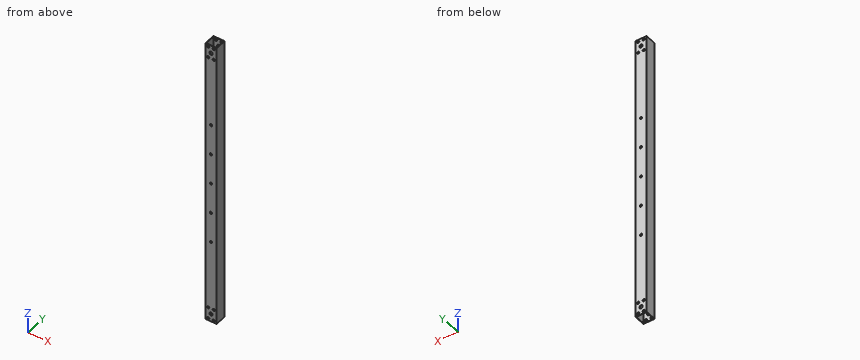
```python
from build123d import *

# Parameters (mm, degrees)
SKETCH_1_W          = 20
SKETCH_1_H          = 20
SKETCH_1_W_2        = 18
SKETCH_1_H_2        = 18
EXTRUDE_1_DEPTH     = 259.5
SKETCH_2_R          = 2.025
SKETCH_2_R_2        = 3.025
CUT_EXTRUDE_1_DEPTH = 20
SKETCH_3_R          = 2.025
CUT_EXTRUDE_2_DEPTH = 20


with BuildPart() as part:
    # 草图1 → 凸台-拉伸1 (new body, symmetric)
    with BuildSketch(Plane.XY):
        Rectangle(SKETCH_1_W, SKETCH_1_H)
        Rectangle(SKETCH_1_W_2, SKETCH_1_H_2, mode=Mode.SUBTRACT)
    extrude(amount=EXTRUDE_1_DEPTH, both=True)

    # 草图2 → 切除-拉伸1 (cut, symmetric)
    with BuildSketch(Plane(origin=(0, 10, 0), x_dir=(1, 0, 0), z_dir=(0, 1, 0))):
        with Locations((-5, 255.5)):
            Circle(SKETCH_2_R)
        with Locations((5, 255.5)):
            Circle(SKETCH_2_R)
        with Locations((-5, 235.5)):
            Circle(SKETCH_2_R)
        with Locations((5, 235.5)):
            Circle(SKETCH_2_R)
        with Locations((0, 245.5)):
            Circle(SKETCH_2_R_2)
        with Locations((5, -235.5)):
            Circle(SKETCH_2_R)
        with Locations((-5, -235.5)):
            Circle(SKETCH_2_R)
        with Locations((-5, -255.5)):
            Circle(SKETCH_2_R)
        with Locations((0, -245.5)):
            Circle(SKETCH_2_R_2)
        with Locations((5, -255.5)):
            Circle(SKETCH_2_R)
    extrude(amount=CUT_EXTRUDE_1_DEPTH, both=True, mode=Mode.SUBTRACT)

    # 草图3 → 切除-拉伸2 (cut)
    with BuildSketch(Plane(origin=(0, 10, 0), x_dir=(1, 0, 0), z_dir=(0, 1, 0))):
        with Locations((0, 110)):
            Circle(SKETCH_3_R)
        with Locations((0, 55)):
            Circle(SKETCH_3_R)
        Circle(SKETCH_3_R)
        with Locations((0, -55)):
            Circle(SKETCH_3_R)
        with Locations((0, -110)):
            Circle(SKETCH_3_R)
    extrude(amount=-CUT_EXTRUDE_2_DEPTH, mode=Mode.SUBTRACT)


solid = part.part
```
Source: CAD feature listing. Evaluate the final solid. Frame: model axes, mm. Coordinates: 2 decimals unless noted, no trailing zeros. Loops run counter-clockwise (first coordinate to the right, second up) from the corner with the lowest first, then second, coordinate; pieces in that order, holes last. Notation, with made-up numbers: M 7.25,42.25 L 45.25,42.25 A14 ccw 45.25,51.25 Z; hole C -1.5,-18.5 d6. An arc over 180 degrees is marked long. Use a Markdown table: item, result. Add a question column.
Q1. Section query B-B, the plane z = 11. Return loops of the section in (x, y), and give its area (3 significant figures).
Q2. Material intervals for L1, parallel to X at y = -7, z = 91; L2, parallel to Z at x = -5, y = 9.3 (3 decimals), sorted ascending.
Q3. Section query A-A, the plane y = 2. Return loops of the section in (x, z), and give its area (3 significant figures).
Result:
| question | item | result |
|---|---|---|
| 1 | outline | M -10,-10 L 10,-10 L 10,10 L -10,10 Z; hole M -9,-9 L 9,-9 L 9,9 L -9,9 Z |
| 1 | area | 76.0 mm2 |
| 2 | L1 | x = -10 to -9, 9 to 10 |
| 2 | L2 | z = -259.5 to -257.525, -253.475 to -237.525, -233.475 to 233.475, 237.525 to 253.475, 257.525 to 259.5 |
| 3 | outline | M -10,-259.5 L -9,-259.5 L -9,259.5 L -10,259.5 Z; M 9,-259.5 L 10,-259.5 L 10,259.5 L 9,259.5 Z |
| 3 | area | 1,040 mm2 |
